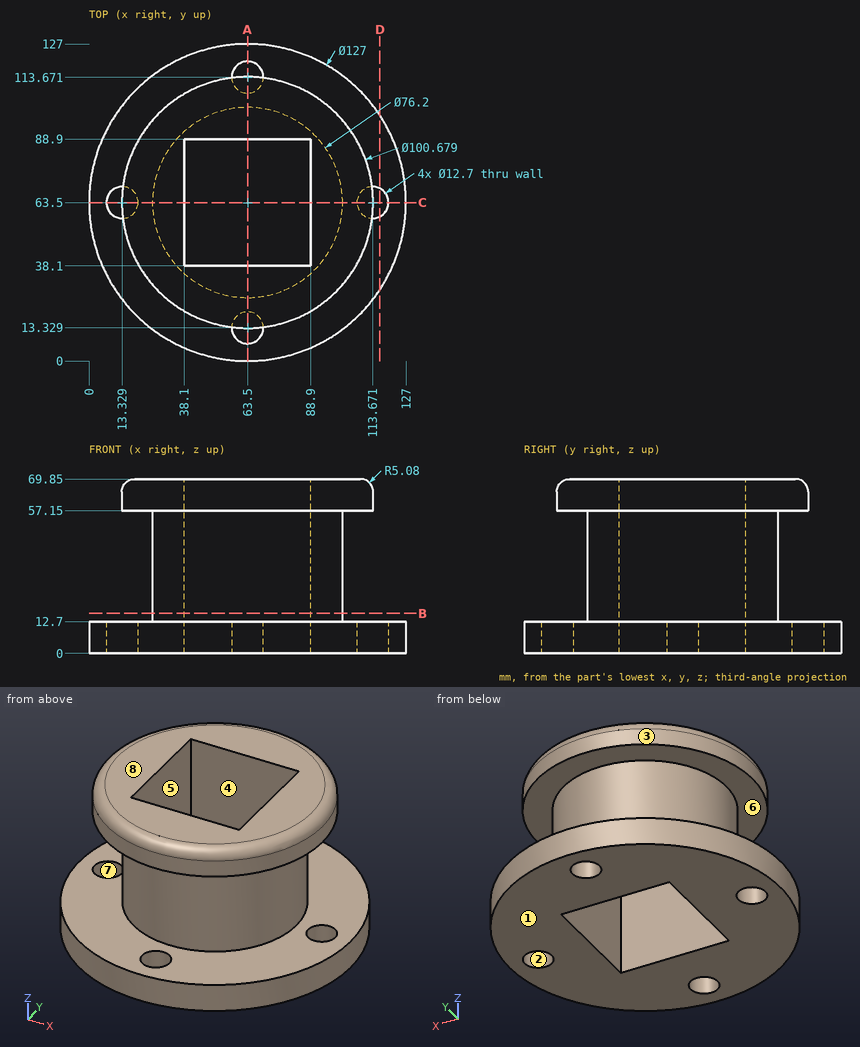
Geometry check sheet. Reference: drawing and pictorial views, mm from the part's lowest x, y, z. A direction names the side the tool comes from. Give positions to 0.01 mm unless a question says otherwise; leave off trailing zeros. Order: outer loops, then holes, each group sorted by start corner. A loop starts at its lowest first (then second) coordinate and runs counter-clockwise, first axis right, second up.
1. Gauge pin test, flat ends, axial feed: pin 1 Ø11.5 at (x, y) = (63.5, 13.33) entering from +Z; pin 2 Ø3 at (x, z) = (89, 31.5) entering from +Y; pin 3 Ø4 at (y, z) = (81, 51.5) entering from +X (1 decimal); pin 4 Ø5 at (y, z) = (30.5, 29.5) entering from -X (1 decimal). Record the tip position at first contact, or that the pin passes through.
2. Access from +Z, -Z, +X, -X, +Y, -Y to the whole of each face (thin tool, end or side, straight path). Record for the marked faces 5, 6, 7 and 8.
3. Release check for a two-part mould opening along Y. For the marked faces 1, 2, 3 and 4 record: pulls with the +Y half, pulls with the -Y half, needs draft (parallel to the pull), parting line crosses it, or undercut.
4. Section check B-B, the plane z = 16. Enter the section's corners in (x, y), and give its area (3 significant figures).
5. Section check A-A, the plane x = 63.5. Enter the section's corners in (y, z), and give its area (3 significant figures).
6. Section check D-D, the plane x = 116.5. Enter the section's corners in (y, z) (1 decimal), and give its area (3 significant figures).
7. Thickness scan on L1, parallel to Y at x = 63.5, z = 5.5; L2, parallel to X at y = 63, z = 9; L3, parallel to Z at x = 42, y = 103. Record the ranges inside material, lowest first.
Values follow:
1. pin 1: stops at z = 69.85
1. pin 2: stops at y = 93.09
1. pin 3: stops at x = 98.3
1. pin 4: stops at x = 40.7
2. face 5: +Z, -Z
2. face 6: none
2. face 7: -Z
2. face 8: +Z, +X, -X, +Y, -Y
3. face 1: needs draft
3. face 2: undercut
3. face 3: parting line crosses it
3. face 4: undercut
4. outline: circle Ø76.2 at (63.5, 63.5); hole (38.1, 38.1) - (88.9, 38.1) - (88.9, 88.9) - (38.1, 88.9) - close
4. area: 1,980 mm2
5. outline: (0, 0) - (6.98, 0) - (6.98, 12.7) - (0, 12.7) - close; (13.16, 57.15) - (25.4, 57.15) - (25.4, 12.7) - (19.68, 12.7) - (19.68, 0) - (38.1, 0) - (38.1, 69.85) - (18.24, 69.85) arc R5.08 ccw to (13.16, 64.77) - close; (88.9, 0) - (107.32, 0) - (107.32, 12.7) - (101.6, 12.7) - (101.6, 57.15) - (113.84, 57.15) - (113.84, 64.77) arc R5.08 ccw to (108.76, 69.85) - (88.9, 69.85) - close; (120.02, 0) - (127, 0) - (127, 12.7) - (120.02, 12.7) - close
5. area: 2,400 mm2
6. outline: (28.5, 0) - (57.8, 0) - (57.8, 12.7) - (28.5, 12.7) - close; (69.2, 0) - (98.5, 0) - (98.5, 12.7) - (69.2, 12.7) - close
6. area: 744 mm2
7. L1: y = 0 to 6.98, 19.68 to 38.1, 88.9 to 107.32, 120.02 to 127
7. L2: x = 0 to 7, 19.66 to 38.1, 88.9 to 107.34, 120 to 127
7. L3: z = 0 to 12.7, 57.15 to 69.85
